Check sheet for the modelled part. Datum: model origin and axes. Units: mm. A direction names the side the tool comes from. Give positions to 0.01 mm unless a question says otherwise; leave off trailing zeros. Loops run counter-clockwise (first coordinate to the right, second up) from the corner with the lowest first, then second, coordinate; pieces in that order, holes last. Notation, with made-up numbers: M 85,18 L 99,18 A27 cw 99,43 Z; hole C 9.5,66 d10. An arc over 180 degrees is marked long. Write each question's results on one line, items separated by ' | '. Start each with the question number.
1. Sectioned sample at D-D on y = -12. Record the cut outline in (x, z) (1 decimal).
2. Sectioned sample at A-A on x = 0. Record the cut outline in (y, z), and give its area (3 significant figures).
3. Material ranges on line 1 along Z through (x, y) = (-6.75, 3.5); line 2 along X through (y, z) = (1.75, -5.5); line 3 along Z through (x, y) = (0, 1.5), recorded low to high.
4. Sectioned sample at C-C on x = -3. Record the cut outline in (y, z).
5. Sectioned sample at B-B on z = 0. Record the cut outline in (x, y).
6. Tool access check on faces 1 (the cylindrical face through (5.245, 3.131, -6.705)), 2 (the flat face through (-4.014, 3.131, 5.698)), 3 (the flat face through (-5.698, 3.131, 4.014)), 4 (the cylindrical face through (5.874, 3.131, 2.413)). Record the directions out of +Z, -Z, +X, -X, +Y, -Y that give a thin tool (end or side, any length) a straight path to the whole face; none if there is none.
7. Go/stop test with flat-tipped pins: pin 1 (6 mm diameter, centred on y = -3.5, z = -2.5, fed in from +X); pin 2 (1.4 mm diameter, centred on y = 4, z = 7, fed in from -X); pin 3 (1.5 mm diameter, centred on x = 1, z = 6.5, fed in from -Y). Record where each tip stops, or that it passes through.
8. Draft check along X on faces 5 (the flat face through (-1.191, 3, -7)), 6 (the cylindrical face through (-5.86, 3.13, 2.45)), 7 (the cylindrical face through (1.026, 3.131, -8.477)), 8 (the flat face through (0, 3, 9.407)). Enter one of: pulls with the +X half, pulls with the -X half, needs draft (parallel to the pull), parting line crosses it, or undercut.
Autodesk Inventor part; units mm, degrees
ref_plane "Work Plane1" through (0, 0, 2.5019) normal (0, 0, 1) x (1, 0, 0)
ref_plane "Work Plane2" through (0, 0, 4.7625) normal (0, 0, 1) x (1, 0, 0)
ref_plane "YZ Plane" through (0, 0, 0) normal (1, 0, 0) x (0, 1, 0)
sketch "Sketch1" plane through (0, 0, 0) normal (0, 1, 0) x (-1, 0, 0)
  line L0 (-7.4806, -1.1906) -> (-6.2374, -1.1906)
  arc A0 (-9.4068, -0.7091) -> (-7.4806, -1.1906) centre (-6.9988, 4.8297) ccw
  line L1 (-9.4068, 0) -> (-9.4068, -0.7091)
  line L2 (-9.4068, 0) -> (-9.4068, 0.7091)
  line L3 (-7.4806, 1.1906) -> (-6.2374, 1.1906)
  arc A1 (-7.4806, 1.1906) -> (-9.4068, 0.7091) centre (-6.9988, -4.8297) ccw
  line L4 (-7.4806, -1.1906) -> (-6.2374, -1.1906)
  arc A2 (-9.4068, -0.7091) -> (-7.4806, -1.1906) centre (-6.9988, 4.8297) ccw
  line L5 (-9.4068, 0) -> (-9.4068, -0.7091)
  line L6 (-9.4068, 0) -> (-9.4068, 0.7091)
  line L7 (-7.4806, 1.1906) -> (-6.2374, 1.1906)
  arc A3 (-7.4806, 1.1906) -> (-9.4068, 0.7091) centre (-6.9988, -4.8297) ccw
  line L8 (-4.4477, -6.1315) -> (-3.5686, -5.2524)
  line L9 (-4.4477, -6.1315) -> (-3.5686, -5.2524)
  line L10 (-6.6516, -6.6516) -> (-6.1502, -7.153)
  line L11 (-6.6516, -6.6516) -> (-6.1502, -7.153)
  line L12 (-6.6516, -6.6516) -> (-7.153, -6.1502)
  line L13 (-6.6516, -6.6516) -> (-7.153, -6.1502)
  line L14 (-6.1315, -4.4477) -> (-5.2524, -3.5686)
  line L15 (-6.1315, -4.4477) -> (-5.2524, -3.5686)
  arc A4 (-6.1315, -4.4477) -> (-7.153, -6.1502) centre (-1.5338, -8.364) ccw
  arc A5 (-6.1315, -4.4477) -> (-7.153, -6.1502) centre (-1.5338, -8.364) ccw
  arc A6 (-6.1502, -7.153) -> (-4.4477, -6.1315) centre (-8.364, -1.5338) ccw
  arc A7 (-6.1502, -7.153) -> (-4.4477, -6.1315) centre (-8.364, -1.5338) ccw
  line L16 (1.1906, -7.4806) -> (1.1906, -6.2374)
  line L17 (1.1906, -7.4806) -> (1.1906, -6.2374)
  line L18 (0, -9.4068) -> (0.7091, -9.4068)
  line L19 (0, -9.4068) -> (0.7091, -9.4068)
  line L20 (0, -9.4068) -> (-0.7091, -9.4068)
  line L21 (0, -9.4068) -> (-0.7091, -9.4068)
  line L22 (-1.1906, -7.4806) -> (-1.1906, -6.2374)
  line L23 (-1.1906, -7.4806) -> (-1.1906, -6.2374)
  arc A8 (-1.1906, -7.4806) -> (-0.7091, -9.4068) centre (4.8297, -6.9988) ccw
  arc A9 (-1.1906, -7.4806) -> (-0.7091, -9.4068) centre (4.8297, -6.9988) ccw
  arc A10 (0.7091, -9.4068) -> (1.1906, -7.4806) centre (-4.8297, -6.9988) ccw
  arc A11 (0.7091, -9.4068) -> (1.1906, -7.4806) centre (-4.8297, -6.9988) ccw
  line L24 (6.1315, -4.4477) -> (5.2524, -3.5686)
  line L25 (6.1315, -4.4477) -> (5.2524, -3.5686)
  line L26 (6.6516, -6.6516) -> (7.153, -6.1502)
  line L27 (6.6516, -6.6516) -> (7.153, -6.1502)
  line L28 (6.6516, -6.6516) -> (6.1502, -7.153)
  line L29 (6.6516, -6.6516) -> (6.1502, -7.153)
  line L30 (4.4477, -6.1315) -> (3.5686, -5.2524)
  line L31 (4.4477, -6.1315) -> (3.5686, -5.2524)
  arc A12 (4.4477, -6.1315) -> (6.1502, -7.153) centre (8.364, -1.5338) ccw
  arc A13 (4.4477, -6.1315) -> (6.1502, -7.153) centre (8.364, -1.5338) ccw
  arc A14 (7.153, -6.1502) -> (6.1315, -4.4477) centre (1.5338, -8.364) ccw
  arc A15 (7.153, -6.1502) -> (6.1315, -4.4477) centre (1.5338, -8.364) ccw
  line L32 (7.4806, 1.1906) -> (6.2374, 1.1906)
  line L33 (7.4806, 1.1906) -> (6.2374, 1.1906)
  line L34 (9.4068, 0) -> (9.4068, 0.7091)
  line L35 (9.4068, 0) -> (9.4068, 0.7091)
  line L36 (9.4068, 0) -> (9.4068, -0.7091)
  line L37 (9.4068, 0) -> (9.4068, -0.7091)
  line L38 (7.4806, -1.1906) -> (6.2374, -1.1906)
  line L39 (7.4806, -1.1906) -> (6.2374, -1.1906)
  arc A16 (7.4806, -1.1906) -> (9.4068, -0.7091) centre (6.9988, 4.8297) ccw
  arc A17 (7.4806, -1.1906) -> (9.4068, -0.7091) centre (6.9988, 4.8297) ccw
  arc A18 (9.4068, 0.7091) -> (7.4806, 1.1906) centre (6.9988, -4.8297) ccw
  arc A19 (9.4068, 0.7091) -> (7.4806, 1.1906) centre (6.9988, -4.8297) ccw
  line L40 (4.4477, 6.1315) -> (3.5686, 5.2524)
  line L41 (4.4477, 6.1315) -> (3.5686, 5.2524)
  line L42 (6.6516, 6.6516) -> (6.1502, 7.153)
  line L43 (6.6516, 6.6516) -> (6.1502, 7.153)
  line L44 (6.6516, 6.6516) -> (7.153, 6.1502)
  line L45 (6.6516, 6.6516) -> (7.153, 6.1502)
  line L46 (6.1315, 4.4477) -> (5.2524, 3.5686)
  line L47 (6.1315, 4.4477) -> (5.2524, 3.5686)
  arc A20 (6.1315, 4.4477) -> (7.153, 6.1502) centre (1.5338, 8.364) ccw
  arc A21 (6.1315, 4.4477) -> (7.153, 6.1502) centre (1.5338, 8.364) ccw
  arc A22 (6.1502, 7.153) -> (4.4477, 6.1315) centre (8.364, 1.5338) ccw
  arc A23 (6.1502, 7.153) -> (4.4477, 6.1315) centre (8.364, 1.5338) ccw
  line L48 (-1.1906, 7.4806) -> (-1.1906, 6.2374)
  line L49 (-1.1906, 7.4806) -> (-1.1906, 6.2374)
  line L50 (0, 9.4068) -> (-0.7091, 9.4068)
  line L51 (0, 9.4068) -> (-0.7091, 9.4068)
  line L52 (0, 9.4068) -> (0.7091, 9.4068)
  line L53 (0, 9.4068) -> (0.7091, 9.4068)
  line L54 (1.1906, 7.4806) -> (1.1906, 6.2374)
  line L55 (1.1906, 7.4806) -> (1.1906, 6.2374)
  arc A24 (1.1906, 7.4806) -> (0.7091, 9.4068) centre (-4.8297, 6.9988) ccw
  arc A25 (1.1906, 7.4806) -> (0.7091, 9.4068) centre (-4.8297, 6.9988) ccw
  arc A26 (-0.7091, 9.4068) -> (-1.1906, 7.4806) centre (4.8297, 6.9988) ccw
  arc A27 (-0.7091, 9.4068) -> (-1.1906, 7.4806) centre (4.8297, 6.9988) ccw
  line L56 (-6.1315, 4.4477) -> (-5.2524, 3.5686)
  line L57 (-6.1315, 4.4477) -> (-5.2524, 3.5686)
  line L58 (-6.6516, 6.6516) -> (-7.153, 6.1502)
  line L59 (-6.6516, 6.6516) -> (-7.153, 6.1502)
  line L60 (-6.6516, 6.6516) -> (-6.1502, 7.153)
  line L61 (-6.6516, 6.6516) -> (-6.1502, 7.153)
  line L62 (-4.4477, 6.1315) -> (-3.5686, 5.2524)
  line L63 (-4.4477, 6.1315) -> (-3.5686, 5.2524)
  arc A28 (-4.4477, 6.1315) -> (-6.1502, 7.153) centre (-8.364, 1.5338) ccw
  arc A29 (-4.4477, 6.1315) -> (-6.1502, 7.153) centre (-8.364, 1.5338) ccw
  arc A30 (-7.153, 6.1502) -> (-6.1315, 4.4477) centre (-1.5338, 8.364) ccw
  arc A31 (-7.153, 6.1502) -> (-6.1315, 4.4477) centre (-1.5338, 8.364) ccw
  arc A32 (1.1906, -6.2374) -> (3.5686, -5.2524) centre (0, 0) ccw
  arc A33 (-3.5686, -5.2524) -> (-1.1906, -6.2374) centre (0, 0) ccw
  arc A34 (-6.2374, -1.1906) -> (-5.2524, -3.5686) centre (0, 0) ccw
  arc A35 (-5.2524, 3.5686) -> (-6.2374, 1.1906) centre (0, 0) ccw
  arc A36 (-1.1906, 6.2374) -> (-3.5686, 5.2524) centre (0, 0) ccw
  arc A37 (3.5686, 5.2524) -> (1.1906, 6.2374) centre (0, 0) ccw
  arc A38 (5.2524, -3.5686) -> (6.2374, -1.1906) centre (0, 0) ccw
  arc A39 (6.2374, 1.1906) -> (5.2524, 3.5686) centre (0, 0) ccw
  point P0 (-6.907, -0.3718)
  point P1 (-6.907, 0.3718)
  point P2 (-6.907, -0.3718)
  point P3 (-6.907, 0.3718)
  point P4 (-4.6211, -5.1469)
  point P5 (-4.6211, -5.1469)
  point P6 (-5.1469, -4.6211)
  point P7 (-5.1469, -4.6211)
  point P8 (0.3718, -6.907)
  point P9 (0.3718, -6.907)
  point P10 (-0.3718, -6.907)
  point P11 (-0.3718, -6.907)
  point P12 (5.1469, -4.6211)
  point P13 (5.1469, -4.6211)
  point P14 (4.6211, -5.1469)
  point P15 (4.6211, -5.1469)
  point P16 (6.907, 0.3718)
  point P17 (6.907, 0.3718)
  point P18 (6.907, -0.3718)
  point P19 (6.907, -0.3718)
  point P20 (4.6211, 5.1469)
  point P21 (4.6211, 5.1469)
  point P22 (5.1469, 4.6211)
  point P23 (5.1469, 4.6211)
  point P24 (-0.3718, 6.907)
  point P25 (-0.3718, 6.907)
  point P26 (0.3718, 6.907)
  point P27 (0.3718, 6.907)
  point P28 (-5.1469, 4.6211)
  point P29 (-5.1469, 4.6211)
  point P30 (-4.6211, 5.1469)
  point P31 (-4.6211, 5.1469)
  dimension "d5" = 360
extrude "Extrusion1" add sketch "Sketch1" along normal blind 6.35
sketch "Sketch2" plane through (0, 0, 0) normal (0, -1, 0) x (1, 0, 0)
  circle A0 centre (0, 0) radius 4.7625
  dimension "d9" = 9.525
extrude "Extrusion2" add sketch "Sketch2" along normal blind 13.97
sketch "Sketch3" plane through (0, 6.35, 0) normal (0, 1, 0) x (1, 0, 0)
  circle A0 centre (0, 0) radius 2.5
  dimension "d12" = 5
extrude "Extrusion3" cut sketch "Sketch3" along normal through all both and the other way through all
ref_plane "Work Plane1" through (0, 0, 2.5019) normal (0, 0, 1) x (1, 0, 0)
ref_plane "Work Plane2" through (0, 0, 4.7625) normal (0, 0, 1) x (1, 0, 0)
sketch "Sketch5" plane through (0, 0, 2.5019) normal (0, 0, 1) x (1, 0, 0)
  line L0 (2.5, -13.97) -> (-2.5, -13.97) construction
  line L1 (0.7091, 6.35) -> (-0.7091, 6.35) construction
  line L2 (0, -13.97) -> (0, -7.62) construction
  circle A0 centre (0, -7.62) radius 2.55
  point P0 (0, 0)
  dimension "d17" = 6.35
  dimension "d18" = 5.1
sketch "Sketch6" plane through (0, 0, 4.7625) normal (0, 0, 1) x (1, 0, 0)
  line L0 (2.5, -13.97) -> (-2.5, -13.97) construction
  line L1 (0, -13.97) -> (0, -7.62) construction
  circle A0 centre (0, -7.62) radius 2.65
  point P0 (0, 0)
  dimension "d19" = 6.35
  dimension "d20" = 5.3
loft "Loft1" cut profiles "Sketch5", "Sketch6"
properties part number "Small Gear"
Output values:
1) outline: C 0,0 d9.5; hole C 0,0 d5
2) outline: M -13.97,-4.76 L 0,-4.76 L 0,-9.41 L 6.35,-9.41 L 6.35,-2.5 L -13.97,-2.5 Z; M -13.97,2.5 L 6.35,2.5 L 6.35,9.41 L 0,9.41 L 0,4.76 L -4.97,4.76 L -5.07,2.5 L -10.17,2.5 L -10.27,4.76 L -13.97,4.76 Z | area: 139 mm2
3) line 1: -6.55 to -5.32, -1.19 to 1.19, 5.32 to 6.55 | line 2: -6.85 to -3.82, -3.17 to 3.17, 3.82 to 6.85 | line 3: -9.41 to -2.5, 2.5 to 9.41
4) outline: M -13.97,-3.7 L 0,-3.7 L 0,-5.6 L 6.35,-5.6 L 6.35,5.6 L 0,5.6 L 0,3.7 L -13.97,3.7 Z
5) outline: M -9.41,0 L -4.76,0 L -4.76,-13.97 L -2.5,-13.97 L -2.5,6.35 L -9.41,6.35 Z; M 2.5,-13.97 L 4.76,-13.97 L 4.76,0 L 9.41,0 L 9.41,6.35 L 2.5,6.35 Z
6) face 1: -Z, +Y, -Y | face 2: +Z, +Y, -Y | face 3: -X, +Y, -Y | face 4: +X, +Y, -Y
7) pin 1: x = 4.76 | pin 2: x = -7 | pin 3: y = 0
8) face 5: undercut | face 6: pulls with the -X half | face 7: pulls with the +X half | face 8: needs draft
